Can you work these out from the model? Positions are in its coordinate system, mm. A direction names the side the tool comes from. Give positions to 0.01 mm unless a question says otherwise; leave off trailing zeros. Order: outer loops, then holes, each group sorted by start corner. A loop starts at its lowest first (then second) coordinate and runs counter-clockwise, first axis right, second up. Notation, with made-up numbers: (-23, -9) -> (28, -9) arc R20 cw to (28, 15) -> close; hole circle Ø5 at (14.25, 40.25). An arc over 180 degrees is marked (long way). Answer as a JSON object with one key per item and string values.
```python
from build123d import *

# Parameters (mm, degrees)
SKETCH1_R           = 47
BOSS_EXTRUDE1_DEPTH = 2
SKETCH3_R           = 2.5
CUT_EXTRUDE1_DEPTH  = 67.498120274
BOSS_EXTRUDE2_DEPTH = 40
CUT_EXTRUDE3_REACH  = 118.892
SKETCH8_R           = 3.25
SKETCH8_R_2         = 2.25
SKETCH9_W           = 11
SKETCH9_H           = 13
CUT_EXTRUDE4_DEPTH  = 1
CUT_EXTRUDE5_DEPTH  = 6


with BuildPart() as part:
    # Sketch1 → Boss-Extrude1 (new body)
    with BuildSketch(Plane.XY):
        Circle(SKETCH1_R)
    extrude(amount=BOSS_EXTRUDE1_DEPTH)

    # Sketch3 → Cut-Extrude1 (cut, through all)
    with BuildSketch(Plane(origin=(0, 0, 0), x_dir=(-1, 0, 0), z_dir=(0, 0, -1))):
        with Locations((30.405591591, 30.405591591)):
            Circle(SKETCH3_R)
        with Locations((11.129218939, -41.53481053)):
            Circle(SKETCH3_R)
        with Locations((-41.53481053, 11.129218939)):
            Circle(SKETCH3_R)
    extrude(amount=-CUT_EXTRUDE1_DEPTH, mode=Mode.SUBTRACT)

    # Sketch4 → Boss-Extrude2 (add)
    with BuildSketch(Plane.XY.offset(2)):
        Polygon((4.020989493, 46.827680313), (32.287890293, 34.153947655), (28.605815439, 25.941620045), (0.338914639, 38.615352703), align=None)
    extrude(amount=BOSS_EXTRUDE2_DEPTH)

    # Sketch8 → Cut-Extrude3 (cut, up to next)
    with BuildSketch(Plane(origin=(18.154439893, 40.490813984, 0), x_dir=(0.9124808455439009, -0.4091194281814147, 0), z_dir=(0.4091194281814148, 0.912480845543901, 0)), mode=Mode.PRIVATE) as cut_extrude3_sk1:
        with Locations(Location((7, -12, 0), (0, 0, 180))):
            Circle(SKETCH8_R)
    cut_extrude3_tool1 = extrude(cut_extrude3_sk1.sketch, amount=-CUT_EXTRUDE3_REACH, mode=Mode.PRIVATE) & part.part
    # Sketch8 → Cut-Extrude3 (cut, up to next)
    with BuildSketch(Plane(origin=(18.154439893, 40.490813984, 0), x_dir=(0.9124808455439009, -0.4091194281814147, 0), z_dir=(0.4091194281814148, 0.912480845543901, 0)), mode=Mode.PRIVATE) as cut_extrude3_sk2:
        with Locations(Location((-7, -12, 0), (0, 0, 180))):
            Circle(SKETCH8_R)
    cut_extrude3_tool2 = extrude(cut_extrude3_sk2.sketch, amount=-CUT_EXTRUDE3_REACH, mode=Mode.PRIVATE) & part.part
    # Sketch8 → Cut-Extrude3 (cut, up to next)
    with BuildSketch(Plane(origin=(18.154439893, 40.490813984, 0), x_dir=(0.9124808455439009, -0.4091194281814147, 0), z_dir=(0.4091194281814148, 0.912480845543901, 0)), mode=Mode.PRIVATE) as cut_extrude3_sk3:
        with Locations(Location((8, -24, 0), (0, 0, 180))):
            Circle(SKETCH8_R_2)
    cut_extrude3_tool3 = extrude(cut_extrude3_sk3.sketch, amount=-CUT_EXTRUDE3_REACH, mode=Mode.PRIVATE) & part.part
    # Sketch8 → Cut-Extrude3 (cut, up to next)
    with BuildSketch(Plane(origin=(18.154439893, 40.490813984, 0), x_dir=(0.9124808455439009, -0.4091194281814147, 0), z_dir=(0.4091194281814148, 0.912480845543901, 0)), mode=Mode.PRIVATE) as cut_extrude3_sk4:
        with Locations(Location((-8, -24, 0), (0, 0, 180))):
            Circle(SKETCH8_R_2)
    cut_extrude3_tool4 = extrude(cut_extrude3_sk4.sketch, amount=-CUT_EXTRUDE3_REACH, mode=Mode.PRIVATE) & part.part
    add(cut_extrude3_tool1.solids().sort_by_distance((24.541806, 37.626978, 12))[0], mode=Mode.SUBTRACT)
    add(cut_extrude3_tool2.solids().sort_by_distance((11.767074, 43.35465, 12))[0], mode=Mode.SUBTRACT)
    add(cut_extrude3_tool3.solids().sort_by_distance((25.454287, 37.217859, 24))[0], mode=Mode.SUBTRACT)
    add(cut_extrude3_tool4.solids().sort_by_distance((10.854593, 43.763769, 24))[0], mode=Mode.SUBTRACT)

    # Sketch9 → Cut-Extrude4 (cut)
    with BuildSketch(Plane(origin=(14.472365039, 32.278486374, 0), x_dir=(0.9124808455439007, -0.40911942818141506, 0), z_dir=(-0.40911942818141506, -0.9124808455439007, 0))):
        with Locations((-7, 12)):
            Rectangle(SKETCH9_W, SKETCH9_H)
        with Locations((7, 12)):
            Rectangle(SKETCH9_W, SKETCH9_H)
    extrude(amount=-CUT_EXTRUDE4_DEPTH, mode=Mode.SUBTRACT)

    # Sketch10 → Cut-Extrude5 (cut)
    with BuildSketch(Plane(origin=(14.472365039, 32.278486374, 0), x_dir=(0.9124808455439007, -0.40911942818141506, 0), z_dir=(-0.40911942818141506, -0.9124808455439007, 0))):
        with BuildLine():
            Line((5.25, 25.198957881), (5.25, 22.801042119))
            ThreePointArc((5.25, 22.801042119), (11, 24), (5.25, 25.198957881))
        make_face()
        with BuildLine():
            Line((-5.25, 25.198957881), (-5.25, 22.801042119))
            ThreePointArc((-5.25, 22.801042119), (-11, 24), (-5.25, 25.198957881))
        make_face()
    extrude(amount=-CUT_EXTRUDE5_DEPTH, mode=Mode.SUBTRACT)


solid = part.part
```
1. If we section it at A-A on z = 10.5: Please give me the cut outline in (x, y), then the cut area to 3 significant figures.
Worked answers:
{"outline": "(0.34, 38.62) -> (3.07, 37.39) -> (3.48, 38.3) -> (5.86, 37.23) -> (9.14, 44.53) -> (4.02, 46.83) -> close; (11.12, 34.88) -> (13.51, 33.8) -> (13.1, 32.89) -> (15.84, 31.66) -> (16.25, 32.58) -> (18.64, 31.51) -> (21.91, 38.81) -> (14.4, 42.18) -> close; (23.9, 29.15) -> (26.29, 28.08) -> (25.88, 27.16) -> (28.61, 25.94) -> (32.29, 34.15) -> (27.17, 36.45) -> close", "area": "165 mm²"}
2. Will these pins go through, and if not, where does the flat tip stop? pin 1 Ø10 at (x, y) = (17, -25.5) entering from +Z; pin 2 Ø4.5 at (x, y) = (7, 36.5) entering from -Z; pin 3 Ø3 at (x, y) = (-30.41, 30.41) entering from +Z; pin 4 Ø3 at (x, z) = (14.5, 32) entering from +Y.
Worked answers:
{"pin 1": "z = 2", "pin 2": "z = 0", "pin 3": "through", "pin 4": "y = 42.8"}
3. If we section it at C-C on y = 0: Please give me the cut outline in (x, z), then the cut area to 3 significant figures.
Worked answers:
{"outline": "(-47, 0) -> (47, 0) -> (47, 2) -> (-47, 2) -> close", "area": "188 mm²"}
4. If we section it at B-B on z = 34: Please give me the cut outline in (x, y), then the cut area to 3 significant figures.
Worked answers:
{"outline": "(0.34, 38.62) -> (28.61, 25.94) -> (32.29, 34.15) -> (4.02, 46.83) -> close", "area": "279 mm²"}
5. For faces 1 (the face through (39.225, 10.172, 0.986)), 2 (the face through (7.801, 41.845, 25.375)), 3 (the face through (17.96, 40.58, 21.72)), which set-ups out of +Z, -Z, +X, -X, +Y, -Y let a thin tool reach every point of the face, with its end or its side?
Worked answers:
{"face 1": "+Z, -Z", "face 2": "none", "face 3": "+Z, +X, +Y"}
6. Please list where these lines run through material, in increasing order: L1, parallel to Z at x = 22, y = 32; L2, parallel to Z at x = -25.5, y = 37; L3, parallel to X at y = 28.5, z = 19.
Worked answers:
{"L1": "0 to 8.75, 15.25 to 21.18, 26.82 to 42", "L2": "0 to 2", "L3": "22.9 to 29.75"}
7. If we mould it in two halves opening along Z, with no side actions, what happens to faces 4 (the face through (21, 30, 18.5)), 5 (the face through (18, 41, 2)), 6 (the face through (30.473, 30.105, 21.72))? For each: +Z half, -Z half, draft (parallel to the pull), parting line (faces both ways), or undercut.
Worked answers:
{"face 4": "undercut", "face 5": "+Z half", "face 6": "draft"}
